from build123d import *

# Parameters (mm, degrees)
F0_R     = 24.5
F1_DEPTH = 5
F2_R     = 37.5
F2_R_2   = 24.5
F3_DEPTH = 5
F4_SIZE  = 1
F5_SIZE  = 1


with BuildPart() as f1:
    # F0 (on Top) → F1 (new body)
    with BuildSketch(Plane.XY):
        Circle(F0_R)
    extrude(amount=F1_DEPTH)

    # F2 (on face) → F3 (join)
    with BuildSketch(Plane.XY.offset(5)):
        Circle(F2_R)
        Circle(F2_R_2, mode=Mode.SUBTRACT)
        Circle(F2_R_2)
    extrude(amount=F3_DEPTH)

    # F4
    f4_edges = [f1.edges().sort_by_distance(p)[0] for p in [
        (-37.5, 0, 10),
    ]]
    chamfer(f4_edges, length=F4_SIZE)

    # F5
    f5_edges = [f1.edges().sort_by_distance(p)[0] for p in [
        (-24.5, 0, 0),
    ]]
    chamfer(f5_edges, length=F5_SIZE)


solid = f1.part
Geometry check sheet. Reference: the model listing, model coordinates, mm. A direction names the side the tool comes from. Coordinates: 2 decimals unless noted, no trailing zeros. Order: outer loops, then holes, each group sorted by start corner. A loop starts at its lowest first (then second) coordinate and runs counter-clockwise, first axis right, second up. Notation, with made-up numbers: (-33.5, 0.25) -> (-12.5, 0.25) arc R12 cw to (-12.5, 17.25) -> close; hole circle Ø9 at (-25.75, 6.25). An arc over 180 degrees is marked (long way). Use a Markdown table: item, result. Add a question column.
1. Set-up check for faces 1 (the face through (13.17, 20.66, 2.97)), 2 (the face through (0, 0, 0)): record each of +Z, -Z, +X, -X, +Y, -Y from which the full face is reachable in a straight line by a thin tool's end or side.
2. Cross-section at C-C (z = 7.75). Enter the section's corners in (x, y).
3. Cross-section at A-A (x = 0). Enter the section's corners in (y, z), and give its area (3 significant figures).
4. Cross-section at D-D (z = 4). Enter the section's corners in (x, y), and give its area (3 significant figures).
5. Go/stop test with flat-tipped pins: pin 1 Ø1.5 at (x, z) = (-24.5, 8.5) entering from +Y; pin 2 Ø3 at (y, z) = (4, 4.5) entering from -X; pin 3 Ø6 at (x, z) = (13, 3) entering from +Y. Record where each tip stops, or that it passes through.
6. Material ranges on L1, parallel to Z at x = 26, y = 14; L2, parallel to X at y = 18, z = 2; L3, parallel to X at y = 6, z = 2.5, recorded low to high.
Filled sheet:
| question | item | result |
|---|---|---|
| 1 | face 1 | -Z |
| 1 | face 2 | -Z, +X, -X, +Y, -Y |
| 2 | outline | circle Ø75 at (0, 0) |
| 3 | outline | (-37.5, 5) -> (-24.5, 5) -> (-24.5, 1) -> (-23.5, 0) -> (23.5, 0) -> (24.5, 1) -> (24.5, 5) -> (37.5, 5) -> (37.5, 9) -> (36.5, 10) -> (-36.5, 10) -> (-37.5, 9) -> close |
| 3 | area | 618 mm2 |
| 4 | outline | circle Ø49 at (0, 0) |
| 4 | area | 1,890 mm2 |
| 5 | pin 1 | y = 29.02 |
| 5 | pin 2 | x = -37.41 |
| 5 | pin 3 | y = 35.92 |
| 6 | L1 | 5 to 10 |
| 6 | L2 | -16.62 to 16.62 |
| 6 | L3 | -23.75 to 23.75 |
